The figure shows three views and two pictorial views of one solid part (mm, origin at its lowest corner). Answer the questions. Give positions to 0.01 mm unless a question says otherwise; leave off trailing zeros. Write each loop counter-clockwise with the first axis right and the second up, starting at its lowest first coordinate (ties: lowest second). Pieces come first, ordered by that corner, then holes. Notation, with made-up numbers: (13, -26) - (39, -26) arc R14 ccw to (39, -1) - close; hole circle Ø4 at (16.5, 66). An arc over 180 degrees is marked (long way). One line per question, with ' | ' between items. Start each with the question number.
1. Find the intervals of material crossed by L1, parallel to Y at x = 18, z = 1.75, in increasing order. Write a range as from..to.
2. A cutting plane is placed at A-A (z = 12.25). Determine the outline of the cut face in (x, y).
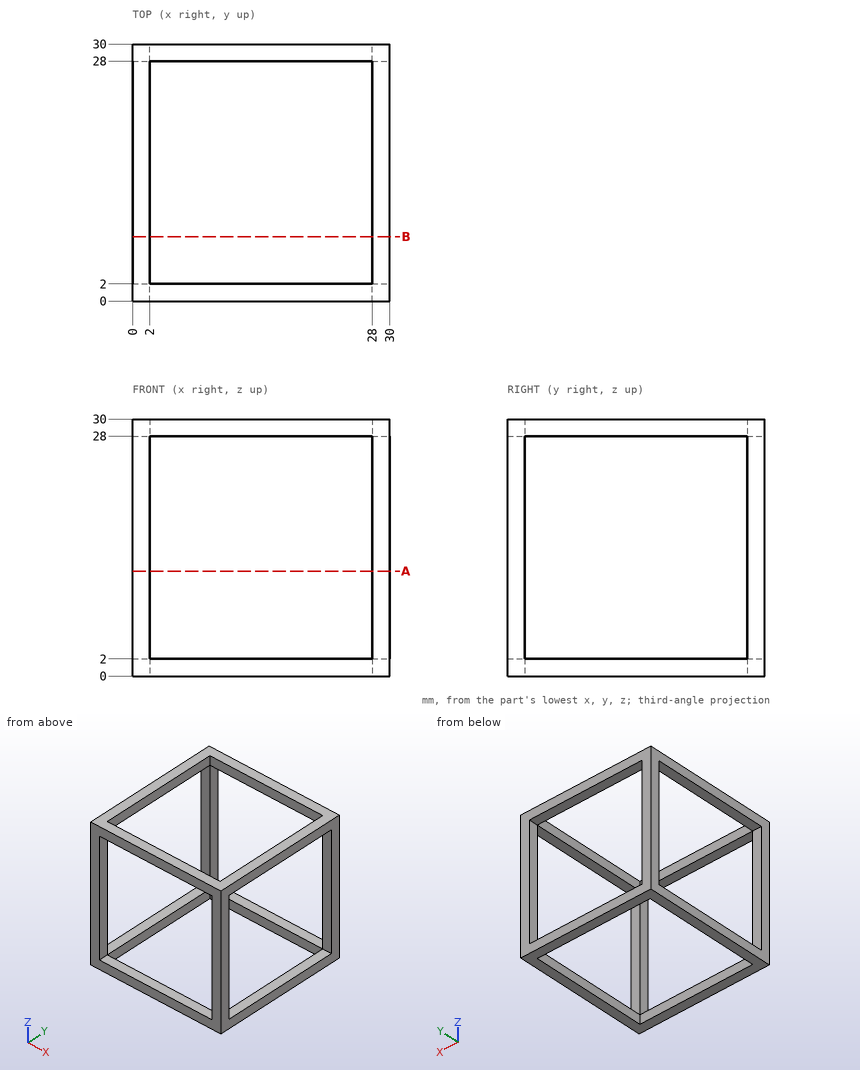
Determined:
1) L1: 0..2, 28..30
2) outline: (0, 0) - (2, 0) - (2, 2) - (0, 2) - close; (0, 28) - (2, 28) - (2, 30) - (0, 30) - close; (28, 0) - (30, 0) - (30, 2) - (28, 2) - close; (28, 28) - (30, 28) - (30, 30) - (28, 30) - close
